```python
from build123d import *

# Parameters (mm, degrees)
F1_DEPTH       = 3
F2_D           = 3.8
F2_CSINK_D     = 6
F2_CSINK_ANGLE = 90
F4_D           = 3.8
F4_CSINK_D     = 6
F4_CSINK_ANGLE = 90


with BuildPart() as f1:
    # F0 (on Top) → F1 (new body)
    with BuildSketch(Plane.XY):
        Polygon((0, 0), (15, 15), (-15, 15), align=None)
        Polygon((15, -15), (15, 15), (0, 0), align=None)
        Polygon((0, 0), (-15, 15), (-15, -15), align=None)
        Polygon((-15, -15), (15, -15), (0, 0), align=None)
    extrude(amount=-F1_DEPTH)

    # F2 (through all)
    with Locations(Plane.XY):
        with Locations((-9.343146, 9.343146), (9.343146, 9.343146), (-9.343146, -9.343146), (9.343146, -9.343146)):
            CounterSinkHole(F2_D / 2, F2_CSINK_D / 2, counter_sink_angle=F2_CSINK_ANGLE)

    # F4 (through all)
    with Locations(Plane(origin=(0, 0, -3), x_dir=(1, 0, 0), z_dir=(0, 0, -1))):
        with Locations((-12, 0), (12, 0)):
            CounterSinkHole(F4_D / 2, F4_CSINK_D / 2, counter_sink_angle=F4_CSINK_ANGLE)


solid = f1.part
```
Model file for the job. Use its own axes, mm. Round coordinates to 2 decimals unless told otherwise and drop trailing zeros. Write each loop counter-clockwise with the first axis right and the second up, starting at its lowest first coordinate (ties: lowest second). Pieces come first, ordered by that corner, then holes. Notation, with made-up numbers: (-30.75, 19) -> (-26.75, 19) arc R5 cw to (-26.75, 23) -> close; hole circle Ø1 at (66, -40). An arc over 180 degrees is marked (long way). Answer as CSV lines item,"result".
1. Mould opens along Y. For faces 1 (the face through (0, 0, -3)), 2 (the face through (0, 15, -1)), 3 (the face through (10.245, 0.728, -0.937)) say: +Y half, -Y half, draft (parallel to the pull), parting line (faces both ways), or undercut.
Resolved:
face 1,"draft"
face 2,"+Y half"
face 3,"undercut"
2. Slice it at A-A, the plane z = -0.65. List the corners of the cut face in (x, y), plus the area to 3 significant figures.
Resolved:
outline,"(-15, -15) -> (15, -15) -> (15, 15) -> (-15, 15) -> close; hole circle Ø3.8 at (-12, 0); hole circle Ø4.7 at (-9.34, -9.34); hole circle Ø4.7 at (-9.34, 9.34); hole circle Ø4.7 at (9.34, -9.34); hole circle Ø4.7 at (9.34, 9.34); hole circle Ø3.8 at (12, 0)"
area,"808 mm²"
3. Slice it at B-B, the plane y = -0.5. State how many separate pieces and enclosed holes the cut face has, plus the area to 3 significant figures.
Resolved:
separate pieces,"3"
enclosed holes,"0"
area,"65.5 mm²"
4. Slice it at D-D, the plane z = -2.6. List the corners of the cut face in (x, y), plus the area to 3 significant figures.
Resolved:
outline,"(-15, -15) -> (15, -15) -> (15, 15) -> (-15, 15) -> close; hole circle Ø5.2 at (-12, 0); hole circle Ø3.8 at (-9.34, -9.34); hole circle Ø3.8 at (-9.34, 9.34); hole circle Ø3.8 at (9.34, -9.34); hole circle Ø3.8 at (9.34, 9.34); hole circle Ø5.2 at (12, 0)"
area,"812 mm²"
5. Drill centre lines: line 1 (Y direction, x = 12, z = -0.8); line 2 (X direction, y = 9.25, z = -2.3); line 3 (X direction, y = -8.5, z = -1.5). Where is each one in solid material? Low to high.
Resolved:
line 1,"-15 to -1.9, 1.9 to 15"
line 2,"-15 to -11.24, -7.45 to 7.45, 11.24 to 15"
line 3,"-15 to -11.05, -7.64 to 7.64, 11.05 to 15"
